Here's how the part is built. I have some questions about the finished solid (model axes, mm). A direction names the side the tool comes from. Coordinates: 2 decimals unless noted, no trailing zeros. Write each loop counter-clockwise with the first axis right and the second up, starting at its lowest first coordinate (ties: lowest second). Pieces come first, ordered by that corner, then holes. Notation, with made-up numbers: M 30,-14 L 75,-14 A13 cw 75,-8 Z; hole C 38.5,-7.75 d8. An arc over 180 degrees is marked long. Use a Markdown table: item, result.
```python
from build123d import *

# Parameters (mm, degrees)
SKETCH1_R               = 16.4
SKETCH1_R_2             = 11.4
BOSS_EXTRUDE1_DEPTH     = 101
CUT_EXTRUDE1_DEPTH      = 10.0001
CUT_EXTRUDE1_DEPTH_BACK = 100
SKETCH2_W               = 2
SKETCH2_H               = 49.498063887
BOSS_EXTRUDE2_START     = 5
BOSS_EXTRUDE2_DEPTH     = 5


with BuildPart() as part:
    # Sketch1 → Boss-Extrude1 (new body)
    with BuildSketch(Plane.XY):
        Circle(SKETCH1_R)
        Circle(SKETCH1_R_2, mode=Mode.SUBTRACT)
    extrude(amount=BOSS_EXTRUDE1_DEPTH)

    # Sketch2 → Cut-Extrude1 (cut, two sides: drawn at the far end of the back side and taken through both)
    with BuildSketch(Plane(origin=(0, 0, 0), x_dir=(0, 0, -1), z_dir=(1, 0, 0)).offset(-CUT_EXTRUDE1_DEPTH_BACK)):
        with Locations((-96, 0.830504428)):
            Rectangle(SKETCH2_W, SKETCH2_H)
    extrude(amount=CUT_EXTRUDE1_DEPTH + CUT_EXTRUDE1_DEPTH_BACK, mode=Mode.SUBTRACT)

    # Sketch3 → Boss-Extrude2 (add)
    with BuildSketch(Plane(origin=(0, 0, 0), x_dir=(-1, 0, 0), z_dir=(0, 0, -1)).offset(BOSS_EXTRUDE2_START)):
        with BuildLine():
            Line((13.164725595, 2.5), (16.208331191, 2.5))
            ThreePointArc((16.208331191, 2.5), (16.4, 0), (16.208331191, -2.5))
            Line((16.208331191, -2.5), (13.164725595, -2.5))
            ThreePointArc((13.164725595, -2.5), (13.4, 0), (13.164725595, 2.5))
        make_face()
        with BuildLine():
            Line((-16.208331191, 2.5), (-13.164725595, 2.5))
            ThreePointArc((-13.164725595, 2.5), (-13.4, 0), (-13.164725595, -2.5))
            Line((-13.164725595, -2.5), (-16.208331191, -2.5))
            ThreePointArc((-16.208331191, -2.5), (-16.4, 0), (-16.208331191, 2.5))
        make_face()
    extrude(amount=-BOSS_EXTRUDE2_DEPTH)


solid = part.part
```
1. Which directions (+Z, -Z, +X, -X, +Y, -Y) give clear straight access to the entire face, cutting with the end or side of a thin tool? Please do faces 5 (the face through (-15, -2.5, -3)), 6 (the face through (15.1, -6.4, 47.3)), 7 (the face through (15, 2.5, -3)), 8 (the face through (-13.4, 0, -2.5)), 9 (the face through (-12, 0, 97)).
Answers follow:
| item | result |
|---|---|
| face 5 | -Z, +X, -X, -Y |
| face 6 | +Z, -Z |
| face 7 | -Z, +X, -X, +Y |
| face 8 | -Z |
| face 9 | -X, +Y, -Y |
2. Suppose I cut it at C-C on z = 73. Write out the boundary of the cut face in (x, y), and give its area (3 significant figures).
Answers follow:
| item | result |
|---|---|
| outline | C 0,0 d32.8; hole C 0,0 d22.8 |
| area | 437 mm2 |
3. Will these pins go through, and if not, where does the flat tip stop? pin 1 Ø13 at (x, y) = (-6, 8) entering from -Z; pin 2 Ø2 at (y, z) = (-11, 30) entering from -X; pin 3 Ø0.9 at (x, z) = (14.5, -1.5) entering from -Y.
Answers follow:
| item | result |
|---|---|
| pin 1 | stops at z = 0 |
| pin 2 | stops at x = -13 |
| pin 3 | stops at y = -2.5 |
4. Suppose I cut it at B-B on y = 0. Write out the boundary of the cut face in (x, z).
Answers follow:
| item | result |
|---|---|
| outline | M -16.4,-5 L -13.4,-5 L -13.4,0 L -11.4,0 L -11.4,95 L -16.4,95 Z; M -16.4,97 L -11.4,97 L -11.4,101 L -16.4,101 Z; M 11.4,0 L 13.4,0 L 13.4,-5 L 16.4,-5 L 16.4,101 L 11.4,101 Z |
5. Suppose I cut it at D-D on y = 4.5. Write out the boundary of the cut face in (x, z).
Answers follow:
| item | result |
|---|---|
| outline | M -15.77,0 L -10.47,0 L -10.47,95 L -15.77,95 Z; M -15.77,97 L -10.47,97 L -10.47,101 L -15.77,101 Z; M 10.47,0 L 15.77,0 L 15.77,101 L 10.47,101 Z |
6. Suppose I cut it at A-A on x = 0. Write out the boundary of the cut face in (y, z), and give its area (3 significant figures).
Answers follow:
| item | result |
|---|---|
| outline | M -16.4,0 L -11.4,0 L -11.4,95 L -16.4,95 Z; M -16.4,97 L -11.4,97 L -11.4,101 L -16.4,101 Z; M 11.4,0 L 16.4,0 L 16.4,95 L 11.4,95 Z; M 11.4,97 L 16.4,97 L 16.4,101 L 11.4,101 Z |
| area | 990 mm2 |
7. We'd pull the mould along Z, two halves only. Please class faces 1 (the face through (10, 9, 96)), 2 (the face through (-11.2, -3.4, 101)), 3 (the face through (-15, 2.5, -3)), 4 (the face through (10, -9, 96)): +Z half, -Z half, draft (parallel to the pull), parting line (faces both ways), or undercut.
Answers follow:
| item | result |
|---|---|
| face 1 | undercut |
| face 2 | +Z half |
| face 3 | draft |
| face 4 | undercut |
8. I need wall thicknesses on probe 1 along X at (y, z) = (0, 71); probe 2 along Z at (x, y) = (7, 13.5); probe 3 along Y at (x, z) = (-10, 7.5). Which ranges of each line are inside material? Lowest first, please.
Answers follow:
| item | result |
|---|---|
| probe 1 | x = -16.4 to -11.4, 11.4 to 16.4 |
| probe 2 | z = 0 to 95, 97 to 101 |
| probe 3 | y = -13 to -5.47, 5.47 to 13 |
